from build123d import *

# Parameters (mm, degrees)
SKETCH1_R           = 50
BOSS_EXTRUDE1_DEPTH = 50
FILLET1_START       = -120
FILLET1_DEPTH       = 240
FILLET1_2_ANGLE     = 180
FILLET1_3_ANGLE     = 180


with BuildPart() as part:
    # Sketch1 → Boss-Extrude1 (new, symmetric)
    with BuildSketch(Plane.XY):
        with BuildLine():
            Line((-65, 55), (65, 55))
            ThreePointArc((65, 55), (120, 0), (65, -55))
            Line((65, -55), (-65, -55))
            ThreePointArc((-65, -55), (-120, 0), (-65, 55))
        make_face()
        with Locations(Location((-65, 0, 0), (0, 0, 180))):
            Circle(SKETCH1_R, mode=Mode.SUBTRACT)
        with Locations(Location((65, 0, 0), (0, 0, 180))):
            Circle(SKETCH1_R, mode=Mode.SUBTRACT)
        with BuildLine():
            Line((-42.087121525, 50), (42.087121525, 50))
            ThreePointArc((42.087121525, 50), (10, 0), (42.087121525, -50))
            Line((42.087121525, -50), (-42.087121525, -50))
            ThreePointArc((-42.087121525, -50), (-10, 0), (-42.087121525, 50))
        make_face(mode=Mode.SUBTRACT)
    extrude(amount=BOSS_EXTRUDE1_DEPTH, both=True)

    # Fillet1: read off the stored shape, not the designer's step
    # Fillet1 outline → Fillet1 (cut)
    with BuildSketch(Plane.YZ.offset(FILLET1_START)):
        with BuildLine():
            Line((55, -50), (55, -45))
            ThreePointArc((55, -45), (53.535533906, -48.535533906), (50, -50))
            Line((50, -50), (55, -50))
        make_face()
        with BuildLine():
            ThreePointArc((50, 50), (53.535533906, 48.535533906), (55, 45))
            Line((55, 45), (55, 50))
            Line((55, 50), (50, 50))
        make_face()
        with BuildLine():
            Line((-55, -50), (-50, -50))
            ThreePointArc((-50, -50), (-53.535533906, -48.535533906), (-55, -45))
            Line((-55, -45), (-55, -50))
        make_face()
        with BuildLine():
            ThreePointArc((-55, 45), (-53.535533906, 48.535533906), (-50, 50))
            Line((-50, 50), (-55, 50))
            Line((-55, 50), (-55, 45))
        make_face()
    extrude(amount=FILLET1_DEPTH, mode=Mode.SUBTRACT)

    # Fillet1 2 outline → Fillet1 2 (revolve, cut)
    with BuildSketch(Plane(origin=(65, 0, 0), x_dir=(0, -1, 0), z_dir=(-1, 0, 0))):
        with BuildLine():
            ThreePointArc((55, -45), (53.535533906, -48.535533906), (50, -50))
            Line((50, -50), (55, -50))
            Line((55, -50), (55, -45))
        make_face()
        with BuildLine():
            ThreePointArc((50, 50), (53.535533906, 48.535533906), (55, 45))
            Line((55, 45), (55, 50))
            Line((55, 50), (50, 50))
        make_face()
    revolve(axis=Axis((65, 0, 0), (0, 0, 1)), revolution_arc=FILLET1_2_ANGLE, mode=Mode.SUBTRACT)

    # Fillet1 3 outline → Fillet1 3 (revolve, cut)
    with BuildSketch(Plane.YZ.offset(-65)):
        with BuildLine():
            ThreePointArc((55, -45), (53.535533906, -48.535533906), (50, -50))
            Line((50, -50), (55, -50))
            Line((55, -50), (55, -45))
        make_face()
        with BuildLine():
            ThreePointArc((50, 50), (53.535533906, 48.535533906), (55, 45))
            Line((55, 45), (55, 50))
            Line((55, 50), (50, 50))
        make_face()
    revolve(axis=Axis((-65, 0, 0), (0, 0, 1)), revolution_arc=FILLET1_3_ANGLE, mode=Mode.SUBTRACT)


solid = part.part
Verification items for the finished model (mm, model axes). A direction names the side the tool comes from. Give positions to 0.01 mm unless a question says otherwise; leave off trailing zeros. Loops run counter-clockwise (first coordinate to the right, second up) from the corner with the lowest first, then second, coordinate; pieces in that order, holes last. Notation, with made-up numbers: (36.5, -16) - (77.5, -16) arc R15 cw to (77.5, 2) - close; hole circle Ø9 at (-8, 12.5). An arc over 180 degrees is marked (long way). Write each question's results on one line, items separated by ' | '.
1) Sectioned sample at D-D on y = -11.5. Count the separate pieces of the cut face and the enclosed holes in it, plus the area to 3 significant figures.
Solution:
separate pieces: 4 | enclosed holes: 0 | area: 2,030 mm2
2) Sectioned sample at A-A on y = 0. Record the boundary of the cut face in (x, z), plus the area to 3 significant figures.
Solution:
outline: (-120, -45) arc R5 ccw to (-115, -50) - (-115, 50) arc R5 ccw to (-120, 45) - close; (-15, -50) - (-10, -50) - (-10, 50) - (-15, 50) - close; (10, -50) - (15, -50) - (15, 50) - (10, 50) - close; (115, -50) arc R5 ccw to (120, -45) - (120, 45) arc R5 ccw to (115, 50) - close | area: 1,980 mm2
3) Tool access check on faces 1 (the flat face through (1, -50, 1)), 2 (the flat face through (15, 8, -50)). Record the directions out of +Z, -Z, +X, -X, +Y, -Y that give a thin tool (end or side, any length) a straight path to the whole face; none if there is none.
Solution:
face 1: +Z, -Z | face 2: -Z, +X, -X, +Y, -Y
4) Sectioned sample at C-C on z = -35. Record the boundary of the cut face in (x, y).
Solution:
outline: (-65, -55) - (65, -55) arc R55 ccw to (65, 55) - (-65, 55) arc R55 ccw to start; hole circle Ø100 at (-65, 0); hole (-42.09, -50) - (42.09, -50) arc R55 cw to (42.09, 50) - (-42.09, 50) arc R55 cw to start; hole circle Ø100 at (65, 0)
5) Depth check by flat-ended pin: P1, Ø1.5, axis at y = 1, z = 26, coming from the -X side; P2, Ø5, axis at y = 7, z = 22.5, coming from the +X side; P3, Ø10, axis at y = 35.5, z = 24, coming from the -X side. Enter the tip coordinate at first touch or a pass-through.
Solution:
P1: x = -120 | P2: x = 119.82 | P3: x = -110.77
6) Material ranges on L1, parallel to X at y = -22.5, z = -42; L2, parallel to Y at x = -65, z = 19; L3, parallel to Y at x = 23.5, z = 12, recorded low to high. Write a range as from..to.
Solution:
L1: -115.19..-109.65, -20.35..-14.81, 14.81..20.35, 109.65..115.19 | L2: -55..-50, 50..55 | L3: -55..-50, -36.09..-27.89, 27.89..36.09, 50..55
7) Sectioned sample at B-B on x = 2. Record the boundary of the cut face in (y, z), plus the area to 3 significant figures.
Solution:
outline: (-55, -45) arc R5 ccw to (-50, -50) - (-50, 50) arc R5 ccw to (-55, 45) - close; (50, -50) arc R5 ccw to (55, -45) - (55, 45) arc R5 ccw to (50, 50) - close | area: 979 mm2
8) Mould release check, pull along X, two halves, no side actions. Record for faces 3 (the cylindrical face through (-119.987, -1.209, 0.63)), 4 (the flat face through (-1, 55, 1)), 5 (the flat face through (-1, 50, 1)): pulls with the +X half, pulls with the -X half, needs draft (parallel to the pull), parting line crosses it, or undercut.
Solution:
face 3: pulls with the -X half | face 4: needs draft | face 5: undercut
